Build history of the part. All positions in model axes, mm. Face numbers are marked on the shaded views. A direction names the side the tool comes from. Give positions to 0.01 mm unless a question says otherwise; leave off trailing zeros. Return JSON: item names as keys, results as strings. Group by question number.
Q1. Band-saw the part on A-A, the plane z = 0. Count the separate pieces of the cut face and the enclosed holes in it, then the cut area to 3 significant figures.
Q2. Pull direction Z, two halves, no side cores. Call the marked faces 5, 6 and 7: +Z half, -Z half, draft (parallel to the pull), parting line (faces both ways), or undercut.
Q3. Flat gauge pins, fed straight in: pin 1 Ø4 at (x, z) = (-5, 7) entering from +Y; pin 2 Ø23 at (y, z) = (9.73, 29.96) entering from -X; pin 3 Ø0.6 at (x, y) = (2, -8) entering from -Z. Where does each tip first touch, or does it go through?
Q4. Wall check: probe 1 along Y at (x, z) = (0, 0); probe 2 along Y at (x, z) = (-5.5, -11.5) (3 decimals); probe 3 along Z at (x, y) = (6, 0). Give the ranges that are in metal, low to high.
Q5. Tool access for the marked faces 1, 2, 3 and 4: list every direction of +Z, -Z, +X, -X, +Y, -Y with a clear straight run to the whole face (end or side of a thin tool).
from build123d import *

# Parameters (mm, degrees)
SKETCH2_R         = 10
EXTRUDE1_DEPTH    = 10
CIRPATTERN1_COUNT = 5
SKETCH3_W         = 4.5
SKETCH3_H         = 2.3
EXTRUDE2_DEPTH    = 16


with BuildPart() as part:
    # Sketch1 → Revolve1 (revolve)
    with BuildSketch(Plane.XY):
        with BuildLine():
            Line((-7.5, 7.5), (7.5, 7.5))
            Line((7.5, 7.5), (7.5, 17.5))
            Line((7.5, 17.5), (7, 17.5))
            ThreePointArc((7, 17.5), (5.585786438, 18.085786438), (5, 19.5))
            Line((5, 19.5), (5, 43.5))
            ThreePointArc((5, 43.5), (5.585786438, 44.914213562), (7, 45.5))
            Line((7, 45.5), (7.5, 45.5))
            Line((7.5, 45.5), (7.5, 52.5))
            Line((7.5, 52.5), (4.5, 52.5))
            Line((4.5, 52.5), (2.5, 45))
            Line((2.5, 45), (-2.5, 45))
            Line((-2.5, 45), (-4.5, 52.5))
            Line((-4.5, 52.5), (-7.5, 52.5))
            Line((-7.5, 52.5), (-7.5, 45.5))
            Line((-7.5, 45.5), (-7, 45.5))
            ThreePointArc((-7, 45.5), (-5.585786438, 44.914213562), (-5, 43.5))
            Line((-5, 43.5), (-5, 19.5))
            ThreePointArc((-5, 19.5), (-5.585786438, 18.085786438), (-7, 17.5))
            Line((-7, 17.5), (-7.5, 17.5))
            Line((-7.5, 17.5), (-7.5, 7.5))
        make_face()
    revolve(axis=Axis((25.864037296, 0, 0), (-1, 0, 0)))

    # Sketch2 → Extrude1 (cut)
    with BuildSketch(Plane(origin=(5, 0, 0), x_dir=(0, 0, -1), z_dir=(1, 0, 0))):
        with Locations((0, 31.5)):
            Circle(SKETCH2_R)
    extrude1 = extrude(amount=-EXTRUDE1_DEPTH, mode=Mode.SUBTRACT)

    # CirPattern1: Extrude1 ×5 about axis
    cirpattern1_axis = Axis((0, 0, 0), (1, 0, 0))
    for i in range(1, CIRPATTERN1_COUNT):
        add(extrude1.rotate(cirpattern1_axis, i * 360 / CIRPATTERN1_COUNT), mode=Mode.SUBTRACT)

    # Sketch3 → Extrude2 (cut, through all)
    with BuildSketch(Plane(origin=(7.5, 0, 0), x_dir=(0, 0, -1), z_dir=(1, 0, 0))):
        with Locations((0, -8.15)):
            Rectangle(SKETCH3_W, SKETCH3_H)
    extrude(amount=-EXTRUDE2_DEPTH, mode=Mode.SUBTRACT)


solid = part.part
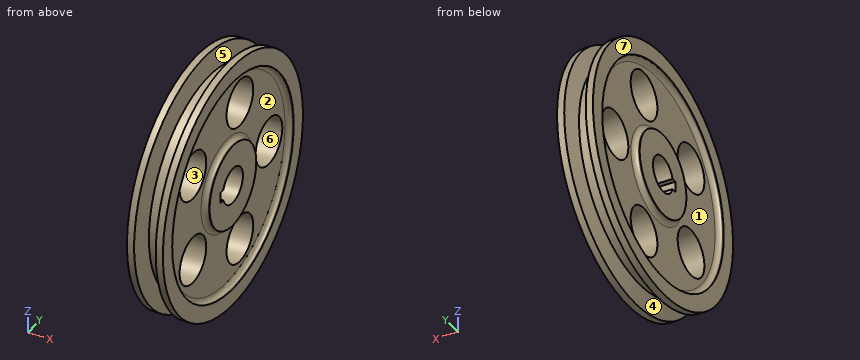
From the geometry:
{
 "1": {"separate pieces": "3", "enclosed holes": "0", "area": "745 mm^2"},
 "2": {"face 5": "parting line", "face 6": "undercut", "face 7": "draft"},
 "3": {"pin 1": "stops at y = 52.26", "pin 2": "stops at x = -5", "pin 3": "stops at z = -44.34"},
 "4": {"probe 1": "y = -45 to -9.3, 7.5 to 21.5, 41.5 to 45", "probe 2": "y = -51.225 to -43.323, -14.077 to 14.077, 43.323 to 51.225", "probe 3": "z = -52.5 to -45.23, -17.77 to -7.5, 7.5 to 17.77, 45.23 to 52.5"},
 "5": {"face 1": "-X", "face 2": "+X", "face 3": "+X, -X", "face 4": "none"}
}
